The listing builds one solid part. Answer for the finished solid, in the listing's coordinates (mm). A direction names the side the tool comes from. Give positions to 0.01 mm unless a question says otherwise; leave off trailing zeros. Write each loop counter-clockwise with the first axis right and the second up, starting at its lowest first coordinate (ties: lowest second). Pieces come first, ordered by that corner, then holes. Notation, with made-up numbers: (-20.5, 18) -> (-13.5, 18) arc R16 cw to (-13.5, 41) -> close; hole circle Ø9 at (36.25, -35). An arc over 180 degrees is marked (long way). One line per question, with ' | ' between items.
from build123d import *

# Parameters (mm, degrees)
SKETCH_1_R      = 5.05
SKETCH_1_R_2    = 2.55
SKETCH_1_W      = 6.2
SKETCH_1_H      = 6.2
EXTRUDE_1_DEPTH = 2


with BuildPart() as part:
    # 草图1 → 凸台-拉伸1 (new body)
    with BuildSketch(Plane.XY):
        with BuildLine():
            Line((0, -25), (36.822908512, -30.548036369))
            Line((36.822908512, -30.548036369), (74.5, -30.548036369))
            Line((74.5, -30.548036369), (74.5, -19))
            Line((74.5, -19), (80.5, -19))
            Line((80.5, -19), (80.5, -11))
            Line((80.5, -11), (74.5, -11))
            Line((74.5, -11), (74.5, -2.05))
            Line((74.5, -2.05), (70.5, -2.05))
            Line((70.5, -2.05), (70.5, -3.5))
            Line((70.5, -3.5), (67.3, -3.5))
            Line((67.3, -3.5), (67.3, -2.05))
            Line((67.3, -2.05), (64.1, -2.05))
            Line((64.1, -2.05), (64.1, 2.05))
            Line((64.1, 2.05), (67.3, 2.05))
            Line((67.3, 2.05), (67.3, 3.5))
            Line((67.3, 3.5), (70.5, 3.5))
            Line((70.5, 3.5), (70.5, 2.05))
            Line((70.5, 2.05), (74.5, 2.05))
            Line((74.5, 2.05), (74.5, 11))
            Line((74.5, 11), (80.5, 11))
            Line((80.5, 11), (80.5, 19))
            Line((80.5, 19), (74.5, 19))
            Line((74.5, 19), (74.5, 30.548036369))
            Line((74.5, 30.548036369), (36.822908512, 30.548036369))
            Line((36.822908512, 30.548036369), (0, 25))
            ThreePointArc((0, 25), (-25, 0), (0, -25))
        make_face()
        Circle(SKETCH_1_R, mode=Mode.SUBTRACT)
        with Locations((55, 5)):
            Circle(SKETCH_1_R_2, mode=Mode.SUBTRACT)
        with Locations(Location((55, -5, 0), (0, 0, 180))):
            Circle(SKETCH_1_R_2, mode=Mode.SUBTRACT)
        with Locations((67.05, -20)):
            Rectangle(SKETCH_1_W, SKETCH_1_H, mode=Mode.SUBTRACT)
        with Locations((49.95, -20)):
            Rectangle(SKETCH_1_W, SKETCH_1_H, mode=Mode.SUBTRACT)
        with Locations((49.95, 20)):
            Rectangle(SKETCH_1_W, SKETCH_1_H, mode=Mode.SUBTRACT)
        with Locations((67.05, 20)):
            Rectangle(SKETCH_1_W, SKETCH_1_H, mode=Mode.SUBTRACT)
    extrude(amount=EXTRUDE_1_DEPTH)


solid = part.part
Item 1: Find section C-C (z = 1.7). Count the separate pieces of the cut face and the enclosed holes in it, then the cut area to 3 significant figures.
Answers below:
separate pieces: 1 | enclosed holes: 7 | area: 5,100 mm²
Item 2: Find section D-D (x = -16). Write down the section's boundary in (y, z).
Answers below:
outline: (-19.21, 0) -> (19.21, 0) -> (19.21, 2) -> (-19.21, 2) -> close
Item 3: Determine the mould class of faces 5 (the face through (27, 0, 0)), 6 (the face through (18.669, 27.813, 0.986)), 7 (the face through (53.05, -20, 1)) for opening direction Y: pulls with the +Y half, pulls with the -Y half, needs draft (parallel to the pull), parting line crosses it, or undercut.
Answers below:
face 5: needs draft | face 6: pulls with the +Y half | face 7: undercut
Item 4: Consider line 1 (Y direction, x = 55, z = 1.3); line 2 (Y direction, x = 47, z = 0.3); line 3 (Y direction, x = 69, z = 1.3). Determine where each line is inside the solid, lowest interval first. Write a range as [from, to].
Answers below:
line 1: [-30.55, -7.55], [-2.45, 2.45], [7.55, 30.55] | line 2: [-30.55, -23.1], [-16.9, 16.9], [23.1, 30.55] | line 3: [-30.55, -23.1], [-16.9, -3.5], [3.5, 16.9], [23.1, 30.55]
Item 5: Find section A-A (x = 55). Write down the section's boundary in (y, z), then the cut area to 3 significant figures.
Answers below:
outline: (-30.55, 0) -> (-7.55, 0) -> (-7.55, 2) -> (-30.55, 2) -> close; (-2.45, 0) -> (2.45, 0) -> (2.45, 2) -> (-2.45, 2) -> close; (7.55, 0) -> (30.55, 0) -> (30.55, 2) -> (7.55, 2) -> close | area: 102 mm²
Item 6: Find section B-B (y = 0). Write down the section's boundary in (x, z), then the cut area to 3 significant figures.
Answers below:
outline: (-25, 0) -> (-5.05, 0) -> (-5.05, 2) -> (-25, 2) -> close; (5.05, 0) -> (64.1, 0) -> (64.1, 2) -> (5.05, 2) -> close | area: 158 mm²
Item 7: Flat-ended cylindrical pins translate along their axes: pin 1 (1 mm diameter, centred on y = -20.5, z = 0.5, fed in from -X); pin 2 (1 mm diameter, centred on x = 76.5, z = 0.5, fed in from -Y); pin 3 (1 mm diameter, centred on y = -5, z = 0.5, fed in from +X). Find the tip coordinate at first contact, or state that the pin passes through.
Answers below:
pin 1: x = -15 | pin 2: y = -19 | pin 3: x = 74.5
Item 8: A tool of negligible diameter and unlimited length cuts with its end or side. For faces 1 (the face through (46.85, 20, 1)), 2 (the face through (77, -19, 1)), 3 (the face through (74.5, 6, 1)), 4 (the face through (78, 19, 1)), from which of +Z, -Z, +X, -X, +Y, -Y can it reach the whole face along a straight path? Write none if from no direction.
Answers below:
face 1: +Z, -Z | face 2: +Z, -Z, +X, -Y | face 3: +Z, -Z, +X | face 4: +Z, -Z, +X, +Y
